The model under review builds one solid part; all positions refer to its coordinate system, in mm. A direction names the side the tool comes from. Coordinates: 2 decimals unless noted, no trailing zeros. Write each loop counter-clockwise with the first axis right and the second up, starting at its lowest first coordinate (ties: lowest second). Pieces come first, ordered by that corner, then holes. Notation, with made-up numbers: (-31, -16.5) -> (-20, -16.5) arc R26 cw to (-20, 1.5) -> close; hole circle Ø9 at (76.5, 43). An arc over 180 degrees is marked (long way). Write each question's results on one line, items separated by ' | '.
```python
from build123d import *

# Parameters (mm, degrees)
F0_W      = 61.3636001945
F0_H      = 59.3294538558
F1_DEPTH  = 30
F1_FACE_W = 61.3636001945
F1_FACE_H = 30
F2_DEPTH  = 20
F2_TAPER  = -3


with BuildPart() as f1:
    # F0 (on Top) → F1 (new body)
    with BuildSketch(Plane.XY):
        with Locations((-38.7336541899, -9.2384442687)):
            Rectangle(F0_W, F0_H)
    extrude(amount=F1_DEPTH)

    # F1_face (on face) → F2 (join)
    with BuildSketch(Plane(origin=(-38.7336541899, -38.9031711966, 15), x_dir=(1, 0, 0), z_dir=(0, -1, 0))):
        Rectangle(F1_FACE_W, F1_FACE_H)
    extrude(amount=F2_DEPTH, taper=F2_TAPER)


solid = f1.part
```
Q1. Clearance check with flat-ended pins moving along their axes: P1, Ø3, axis at y = -17, z = 14.5, coming from the +X side; P2, Ø2, axis at x = -21, y = -38.5, coming from the +Z side; P3, Ø1, axis at x = -34, y = -39.5, coming from the -Z side. State where each tip first meets the part, or that it passes through.
Solution:
P1: x = -8.05 | P2: z = 30.03 | P3: z = -0.06
Q2. For line 1 (X direction, y = -23.5, z = 18.5); line 2 (Z direction, x = -48, y = -1); line 3 (Z direction, x = -48.5, y = -51), list the stretches that pass through material, from the lowest coordinate up. Write a range as from..to.
Solution:
line 1: -69.42..-8.05 | line 2: 0..30 | line 3: -0.63..30.63
Q3. Add section A-A (y = -7). Write out the cut boundary in (x, z).
Solution:
outline: (-69.42, 0) -> (-8.05, 0) -> (-8.05, 30) -> (-69.42, 30) -> close
Q4. Machinability: for faces 1 (the flat face through (-39, -9, 0)), 2 (the flat face through (-8.052, -10, 15)), 3 (the flat face through (-39, -9, 30)), which of the approach directions +Z, -Z, +X, -X, +Y, -Y give a long, thin tool a straight path to every point of the face, cutting with its end or side? Answer none if there is none.
Solution:
face 1: -Z, +X, -X, +Y | face 2: +Z, -Z, +X, +Y | face 3: +Z, +X, -X, +Y
